Design review of the part built by this model. Coordinates are the model's own, in mm. Face numbers are marked on the shaded views. A direction names the side the tool comes from. Coordinates: 2 decimals unless noted, no trailing zeros. Order: outer loops, then holes, each group sorted by start corner. A loop starts at its lowest first (then second) coordinate and runs counter-clockwise, first axis right, second up. Notation, with made-up numbers: M -35,-8.75 L 3,-8.75 A20 cw 3,6.25 Z; hole C 17.5,17 d1. An arc over 180 degrees is marked long. Answer in a Markdown table with one row per item.
from build123d import *

# Parameters (mm, degrees)
F0_W     = 80
F0_H     = 60
F1_DEPTH = 10
F2_R     = 13.3
F3_DEPTH = 10.001
F4_R     = 4
F5_DEPTH = 10.001
F6_R     = 5
F7_W     = 14
F7_H     = 22
F8_DEPTH = 5
F9_R     = 5


with BuildPart() as f1:
    # F0 (on Front) → F1 (new body)
    with BuildSketch(Plane.XZ):
        with Locations((0, 10)):
            Rectangle(F0_W, F0_H)
    extrude(amount=F1_DEPTH)

    # F2 (on face) → F3 (cut, through all)
    with BuildSketch(Plane.XZ.offset(10)):
        with Locations((0, 10)):
            Circle(F2_R)
    extrude(amount=-F3_DEPTH, mode=Mode.SUBTRACT)

    # F4 (on face) → F5 (cut, through all)
    with BuildSketch(Plane.XZ.offset(10)):
        with Locations((-31, 31)):
            Circle(F4_R)
        with Locations((31, 31)):
            Circle(F4_R)
        with Locations((-31, -11)):
            Circle(F4_R)
        with Locations((31, -11)):
            Circle(F4_R)
    extrude(amount=-F5_DEPTH, mode=Mode.SUBTRACT)

    # F6
    f6_edges = [f1.edges().sort_by_distance(p)[0] for p in [
        (40, -5, 40),
        (40, -5, -20),
        (-40, -5, -20),
        (-40, -5, 40),
    ]]
    fillet(f6_edges, radius=F6_R)

    # F7 (on face) → F8 (cut)
    with BuildSketch(Plane.XZ.offset(10)):
        Polygon((-24.5, 34.7527767497), (-31, 38.5055534995), (-37.5, 34.7527767497), (-37.5, 27.2472232503), (-31, 23.4944465005), (-24.5, 27.2472232503), align=None)
        Polygon((24.5, 34.7527767497), (24.5, 27.2472232503), (31, 23.4944465005), (37.5, 27.2472232503), (37.5, 34.7527767497), (31, 38.5055534995), align=None)
        Polygon((24.5, -7.2472232503), (24.5, -14.7527767497), (31, -18.5055534995), (37.5, -14.7527767497), (37.5, -7.2472232503), (31, -3.4944465005), align=None)
        Polygon((-24.5, -7.2472232503), (-31, -3.4944465005), (-37.5, -7.2472232503), (-37.5, -14.7527767497), (-31, -18.5055534995), (-24.5, -14.7527767497), align=None)
        with BuildLine():
            ThreePointArc((13.6106575888, 21), (16.499037969, 15.8336734651), (17.5, 10))
            ThreePointArc((17.5, 10), (16.499037969, 4.1663265349), (13.6106575888, -1))
            Line((13.6106575888, -1), (22, -1))
            Line((22, -1), (22, 21))
            Line((22, 21), (13.6106575888, 21))
        make_face()
        with BuildLine():
            ThreePointArc((-13.6106575888, 21), (0, 27.5), (13.6106575888, 21))
            Line((13.6106575888, 21), (22, 21))
            Line((22, 21), (22, 36))
            Line((22, 36), (-22, 36))
            Line((-22, 36), (-22, 21))
            Line((-22, 21), (-13.6106575888, 21))
        make_face()
        with BuildLine():
            Line((22, -1), (13.6106575888, -1))
            ThreePointArc((13.6106575888, -1), (0, -7.5), (-13.6106575888, -1))
            Line((-13.6106575888, -1), (-22, -1))
            Line((-22, -1), (-22, -16))
            Line((-22, -16), (22, -16))
            Line((22, -16), (22, -1))
        make_face()
        with BuildLine():
            ThreePointArc((-13.6106575888, -1), (-17.5, 10), (-13.6106575888, 21))
            Line((-13.6106575888, 21), (-22, 21))
            Line((-22, 21), (-22, -1))
            Line((-22, -1), (-13.6106575888, -1))
        make_face()
        with Locations((29, 10)):
            Rectangle(F7_W, F7_H)
        with Locations((-29, 10)):
            Rectangle(F7_W, F7_H)
    extrude(amount=-F8_DEPTH, mode=Mode.SUBTRACT)

    # F9
    f9_edges = [f1.edges().sort_by_distance(p)[0] for p in [
        (-22, -7.5, 21),
        (-36, -7.5, 21),
        (-22, -7.5, 36),
        (22, -7.5, 36),
        (22, -7.5, 21),
        (36, -7.5, 21),
        (-36, -7.5, -1),
        (-22, -7.5, -1),
        (-22, -7.5, -16),
        (36, -7.5, -1),
        (22, -7.5, -1),
        (22, -7.5, -16),
    ]]
    fillet(f9_edges, radius=F9_R)


solid = f1.part
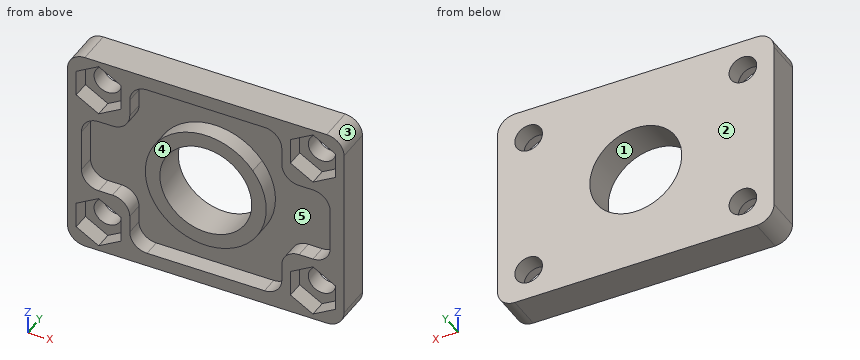
(1) Add section D-D, the plane y = -8. Give the number of separate pieces and of enclosed holes in the cut face, and give its area (3 significant figures).
Return value:
| item | result |
|---|---|
| separate pieces | 2 |
| enclosed holes | 6 |
| area | 1,720 mm2 |
(2) Add section B-B, the plane z = 10. Give the boundary of the cut face in (x, y).
Return value:
| item | result |
|---|---|
| outline | M -40,-10 L -36,-10 L -36,-5 L -17.5,-5 L -17.5,-10 L -13.3,-10 L -13.3,0 L -40,0 Z; M 13.3,-10 L 17.5,-10 L 17.5,-5 L 36,-5 L 36,-10 L 40,-10 L 40,0 L 13.3,0 Z |
(3) For the marked faces 4 and 5, list the 3-axis set-ups (+Z, -Z, +X, -X, +Y, -Y) from which the entire face can be reached by the end or side of a thin tool; tool diameter is ignored.
Return value:
| item | result |
|---|---|
| face 4 | +Z, -Z, +X, -X, -Y |
| face 5 | -Y |
(4) Draft analysis for pull direction X (two halves, no side actions). For the marked faces 1, 2 and 3, state which applies: pulls with the +X half, pulls with the -X half, needs draft (parallel to the pull), parting line crosses it, or undercut.
Return value:
| item | result |
|---|---|
| face 1 | undercut |
| face 2 | needs draft |
| face 3 | pulls with the +X half |
(5) Insertion check: pin 1 Ø2 at (x, z) = (9.5, -11.5) entering from -Y; pin 2 Ø6.5 at (x, z) = (-31, 31) entering from -Y. Each pin has a flat end and moves straight along its axis. Give the tip position at first contact, or say it passes through.
Return value:
| item | result |
|---|---|
| pin 1 | stops at y = -5 |
| pin 2 | passes through |
(6) Add section A-A, the plane x = 0. Give the boundary of the cut face in (y, z), and give its area (3 significant figures).
Return value:
| item | result |
|---|---|
| outline | M -10,-20 L 0,-20 L 0,-3.3 L -10,-3.3 L -10,-7.5 L -5,-7.5 L -5,-16 L -10,-16 Z; M -10,23.3 L 0,23.3 L 0,40 L -10,40 L -10,36 L -5,36 L -5,27.5 L -10,27.5 Z |
| area | 249 mm2 |
(7) Add section C-C, the plane y = -1.5. Give the boundary of the cut face in (x, z).
Return value:
| item | result |
|---|---|
| outline | M -40,-15 A5 ccw -35,-20 L 35,-20 A5 ccw 40,-15 L 40,35 A5 ccw 35,40 L -35,40 A5 ccw -40,35 Z; hole C -31,-11 d8; hole C -31,31 d8; hole C 0,10 d26.6; hole C 31,-11 d8; hole C 31,31 d8 |
(8) For line 1 along X through (y, z) = (-5.5, -11); line 2 along Z through (x, y) = (-31, -3.95); line 3 along Z through (x, y) = (-10, -5.5), list the stretches that pass through material, from the lowest coordinate up. Write a range as from..to.
Return value:
| item | result |
|---|---|
| line 1 | x = -40..-37.5, -24.5..-22, 22..24.5, 37.5..40 |
| line 2 | z = -20..-15, -7..27, 35..40 |
| line 3 | z = -20..-16, -4.36..1.23, 18.77..24.36, 36..40 |
